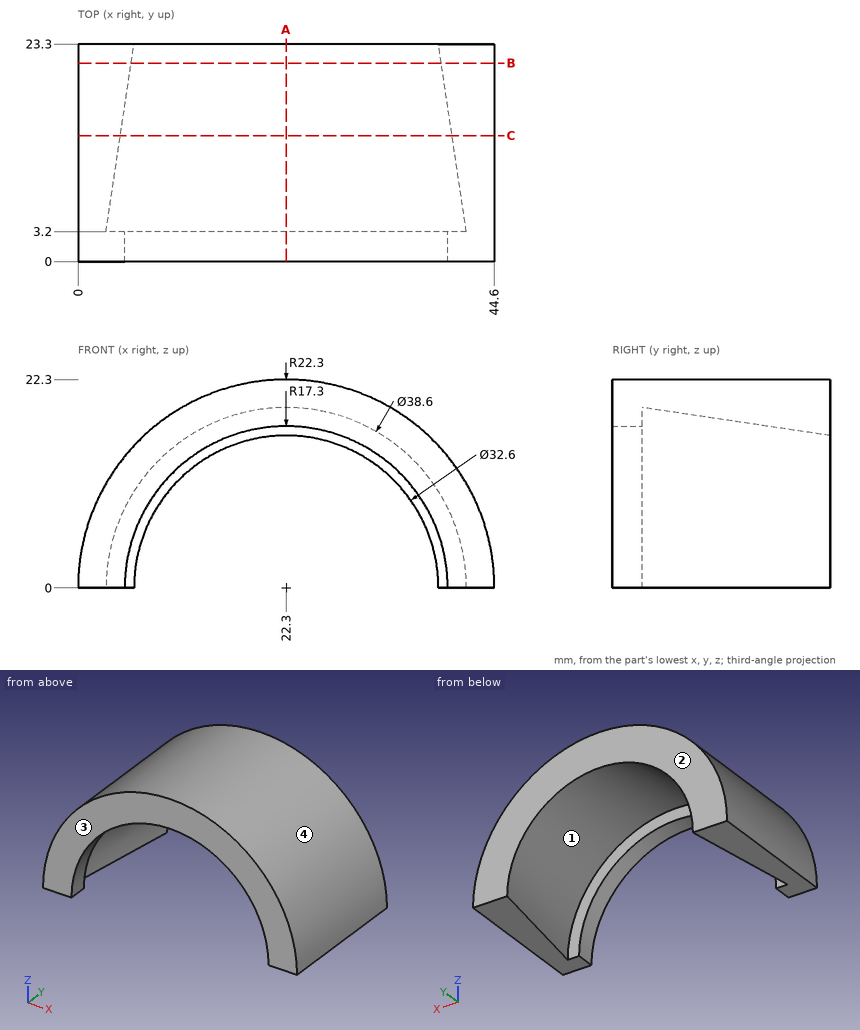
Job drawing, mm, ordinate dimensions from the low corner. One solid piece. Round coordinates to 2 decimals unless told otherwise and drop trailing zeros. Order: outer loops, then holes, each group sorted by start corner. A loop starts at its lowest first (then second) coordinate and runs counter-clockwise, first axis right, second up. Notation, with made-up numbers: (29.25, -18.75) -> (39.25, -18.75) arc R29 cw to (39.25, 11.25) -> close; hole circle Ø7 at (4.5, -16). An arc over 180 degrees is marked (long way). Write item = value, one per line.
(1) Cut at B-B (y = 21.25). Write the cut outline in (x, z).
Answers follow:
outline = (0, 0) -> (5.69, 0) arc R16.61 cw to (38.91, 0) -> (44.6, 0) arc R22.3 ccw to start
(2) Flat gauge pins, fed straight in: P1, Ø6, axis at y = 12, z = 11.5, coming from the +X side; P2, Ø3, axis at x = 8.5, y = 16.5, coming from the +Z side; P3, Ø8, axis at y = 6, z = 16, coming from the -X side. Where does each tip first touch, or does it go through?
Answers follow:
P1 = 42.92
P2 = 18.6
P3 = 3.5
(3) Cut at A-A (x = 22.3). Write the cut outline in (y, z).
Answers follow:
outline = (0, 17.3) -> (3.2, 17.3) -> (3.2, 19.3) -> (23.3, 16.3) -> (23.3, 22.3) -> (0, 22.3) -> close
(4) Drill centre lines: L1, parallel to X at y = 4.5, z = 6.5; L2, parallel to X at y = 16.5, z = 12; L3, parallel to Z at x = 22.5, y = 15.75. Where is each one in solid material? Low to high.
Answers follow:
L1 = 0.97 to 4.33, 40.27 to 43.63
L2 = 3.5 to 9.82, 34.78 to 41.1
L3 = 17.43 to 22.3
(5) Pull direction Y, two halves, no side cores. Call the marked faces 1, 2, 3 and 4: +Y half, -Y half, draft (parallel to the pull), parting line (faces both ways), or undercut.
Answers follow:
face_1 = undercut
face_2 = +Y half
face_3 = -Y half
face_4 = draft
(6) Cut at C-C (y = 13.5). Write the cut outline in (x, z).
Answers follow:
outline = (0, 0) -> (4.54, 0) arc R17.76 cw to (40.06, 0) -> (44.6, 0) arc R22.3 ccw to start
